Work out the finished part from the listing and answer in its coordinate system (mm). Face numbers are marked on the shaded views. A direction names the side the tool comes from. Coordinates: 2 decimals unless noted, no trailing zeros. Loops run counter-clockwise (first coordinate to the right, second up) from the corner with the lowest first, then second, coordinate; pieces in that order, holes last. Notation, with made-up numbers: (59, -14) -> (67, -14) arc R18 ccw to (67, 11) -> close; hole circle Ø4 at (68.5, 65.5). An arc over 180 degrees is marked (long way). Use a Markdown table: item, result. Add a question column.
```python
from build123d import *

# Parameters (mm, degrees)
SKETCH1_W           = 38.350231224
SKETCH1_H           = 38.350231224
BOSS_EXTRUDE1_DEPTH = 5
SKETCH2_W           = 28.750231224
SKETCH2_H           = 28.750231224
BOSS_EXTRUDE2_DEPTH = 20
CHAMFER1_SIZE       = 5
SKETCH3_R           = 2.332714882
SKETCH3_W           = 17.69914949
SKETCH3_H           = 13.531318076
CUT_EXTRUDE1_DEPTH  = 5
SKETCH4_R           = 4.319213653
CUT_EXTRUDE2_DEPTH  = 9


with BuildPart() as part:
    # Sketch1 → Boss-Extrude1 (new body)
    with BuildSketch(Plane(origin=(0, 0, 0), x_dir=(1, 0, 0), z_dir=(0, 1, 0))):
        Rectangle(SKETCH1_W, SKETCH1_H)
    extrude(amount=BOSS_EXTRUDE1_DEPTH)

    # Sketch2 → Boss-Extrude2 (add)
    with BuildSketch(Plane(origin=(0, 0, 0), x_dir=(1, 0, 0), z_dir=(0, 1, 0))):
        Rectangle(SKETCH2_W, SKETCH2_H)
    extrude(amount=-BOSS_EXTRUDE2_DEPTH)

    # Chamfer1
    chamfer1_edges = [part.edges().sort_by_distance(p)[0] for p in [
        (14.375115612, -10, -14.375115612),
        (14.375115612, -10, 14.375115612),
        (-14.375115612, -10, 14.375115612),
        (-14.375115612, -10, -14.375115612),
        (19.175115612, 2.5, 19.175115612),
        (-19.175115612, 2.5, 19.175115612),
        (-19.175115612, 2.5, -19.175115612),
        (19.175115612, 2.5, -19.175115612),
    ]]
    chamfer(chamfer1_edges, length=CHAMFER1_SIZE)

    # Sketch3 → Cut-Extrude1 (cut)
    with BuildSketch(Plane(origin=(0, 5, 0), x_dir=(1, 0, 0), z_dir=(0, 1, 0))):
        with Locations((-12.184831311, 0)):
            Circle(SKETCH3_R)
        with Locations((12.184831311, 0)):
            Circle(SKETCH3_R)
        Rectangle(SKETCH3_W, SKETCH3_H)
    extrude(amount=-CUT_EXTRUDE1_DEPTH, mode=Mode.SUBTRACT)

    # Sketch4 → Cut-Extrude2 (cut)
    with BuildSketch(Plane.XZ.offset(20)):
        Circle(SKETCH4_R)
    extrude(amount=-CUT_EXTRUDE2_DEPTH, mode=Mode.SUBTRACT)


solid = part.part
```
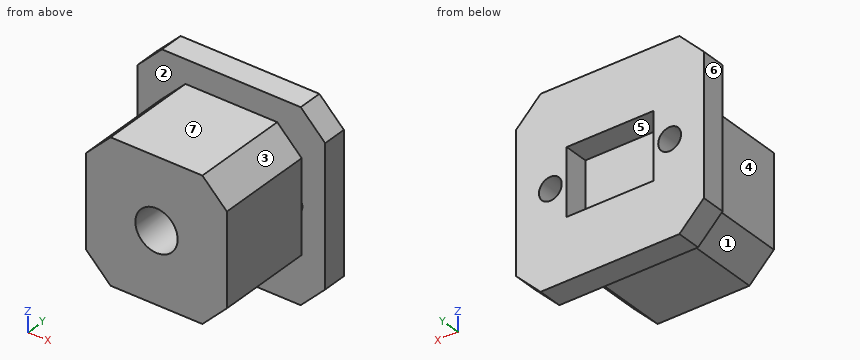
Item 1: Section A-A (z = 0) is taken. Determine the outline of the cut face in (x, y).
Item 2: Given pin 1 (10 mm diameter, centred on y = -12.5, z = 15.5, fed in from -X); pin 2 (1.4 mm diameter, centred on x = -11.5, z = -1, fed in from +Y); pin 3 (10 mm diameter, centred on x = -15, y = -9.5, fed in from -Z), each flat-ended and moving along its own axis, determine where each tip first touches the part or whether it passes through.
Item 3: Find the intervals of material crossed by probe 1 along X at (y, z) = (2.3, 0); probe 2 along Z at (x, y) = (5.5, 2.75); probe 3 along Z at (x, y) = (0, -17.5), in increasing order.
Item 4: For the marked faces 1, 2, 3 and 4, determine the directions among +Z, -Z, +X, -X, +Y, -Y from which every point of the face is accessible in a straight line to the end or side of a thin tool.
Item 5: Section D-D (y = -5.25) is taken. Determine the outline of the cut face in (x, z).
Item 6: For a pull along Z with two mould halves and no side action, classify the marked faces 5, 6 and 7 as +Z half, -Z half, draft (parallel to the pull), parting line (faces both ways), or undercut.
Item 7: Section B-B (y = 1) is taken. Determine the outline of the cut face in (x, z), then the cut area to 3 significant figures.
Item 8: Section C-C (y = -14.75) is taken. Determine the outline of the cut face in (x, z).
Output:
| question | item | result |
|---|---|---|
| 1 | outline | (-19.18, 0) -> (-14.52, 0) -> (-14.52, 5) -> (-19.18, 5) -> close; (-14.38, -20) -> (-4.32, -20) -> (-4.32, -11) -> (4.32, -11) -> (4.32, -20) -> (14.38, -20) -> (14.38, 0) -> (9.85, 0) -> (9.85, 5) -> (8.85, 5) -> (8.85, 0) -> (-8.85, 0) -> (-8.85, 5) -> (-9.85, 5) -> (-9.85, 0) -> (-14.38, 0) -> close; (14.52, 0) -> (19.18, 0) -> (19.18, 5) -> (14.52, 5) -> close |
| 2 | pin 1 | stops at x = -13.25 |
| 2 | pin 2 | stops at y = 0 |
| 2 | pin 3 | stops at z = -13.75 |
| 3 | probe 1 | x = -19.18 to -14.52, -9.85 to -8.85, 8.85 to 9.85, 14.52 to 19.18 |
| 3 | probe 2 | z = -19.18 to -6.77, 6.77 to 19.18 |
| 3 | probe 3 | z = -14.38 to -4.32, 4.32 to 14.38 |
| 4 | face 1 | -Z, -X, -Y |
| 4 | face 2 | -Y |
| 4 | face 3 | +Z, +X, -Y |
| 4 | face 4 | +Z, -Z, -X, -Y |
| 5 | outline | (-14.38, -9.38) -> (-9.38, -14.38) -> (9.38, -14.38) -> (14.38, -9.38) -> (14.38, 9.38) -> (9.38, 14.38) -> (-9.38, 14.38) -> (-14.38, 9.38) -> close |
| 6 | face 5 | undercut |
| 6 | face 6 | draft |
| 6 | face 7 | +Z half |
| 7 | outline | (-19.18, -14.18) -> (-14.18, -19.18) -> (14.18, -19.18) -> (19.18, -14.18) -> (19.18, 14.18) -> (14.18, 19.18) -> (-14.18, 19.18) -> (-19.18, 14.18) -> close; hole circle Ø4.67 at (-12.18, 0); hole (-8.85, -6.77) -> (8.85, -6.77) -> (8.85, 6.77) -> (-8.85, 6.77) -> close; hole circle Ø4.67 at (12.18, 0) |
| 7 | area | 1,150 mm2 |
| 8 | outline | (-14.38, -9.38) -> (-9.38, -14.38) -> (9.38, -14.38) -> (14.38, -9.38) -> (14.38, 9.38) -> (9.38, 14.38) -> (-9.38, 14.38) -> (-14.38, 9.38) -> close; hole circle Ø8.64 at (0, 0) |
